from build123d import *

# Parameters (mm, degrees)
F1_DEPTH      = 25.4
F1_DEPTH_BACK = 25.4


with BuildPart() as f1:
    # F0 (on Front) → F1 (new body, two sides)
    with BuildSketch(Plane.XZ) as f1_sk:
        with BuildLine():
            Line((-8.390563, 22.175057), (-48.245732, 0))
            Line((-48.245732, 0), (-97.690113, -9.289551))
            Line((-97.690113, -9.289551), (-97.690113, -29.067304))
            Line((-97.690113, -29.067304), (-72.518431, -29.067304))
            ThreePointArc((-72.518431, -29.067304), (-57.08579, -12.585117), (-41.653149, -29.067304))
            Line((-41.653149, -29.067304), (38.356856, -29.067304))
            ThreePointArc((38.356856, -29.067304), (50.593399, -7.999803), (61.131231, -29.966293))
            Line((61.131231, -29.966293), (91.397189, -29.966293))
            Line((91.397189, -29.966293), (91.397189, -4.195281))
            Line((91.397189, -4.195281), (65.925851, 0))
            Line((65.925851, 0), (42.098479, 22.175057))
            Line((42.098479, 22.175057), (-8.390563, 22.175057))
        make_face()
    extrude(amount=F1_DEPTH)
    extrude(f1_sk.sketch, amount=-F1_DEPTH_BACK)


solid = f1.part
The listing builds one solid part. Answer for the finished solid, in the listing's coordinates (mm). A direction names the side the tool comes from. Give positions to 0.01 mm unless a question says otherwise; leave off trailing zeros. Loops run counter-clockwise (first coordinate to the right, second up) from the corner with the lowest first, then second, coordinate; pieces in that order, holes last. Notation, with made-up numbers: (13, -8.5) - (55, -8.5) arc R14 ccw to (55, 13.5) - close; hole circle Ø10 at (77, 31.5). An arc over 180 degrees is marked (long way). Answer as a JSON object with one key per item and string values.
1. Find the intervals of material crossed by L1, parallel to X at y = -9.5, z = -22; L2, parallel to X at y = -5, z = -23; L3, parallel to Z at x = 24, y = -13.5, in increasing order. Write a range as [from, to].
Determined:
{"L1": "[-97.69, -71.32], [-42.85, 36.27], [63.83, 91.4]", "L2": "[-97.69, -71.7], [-42.47, 36.32], [63.78, 91.4]", "L3": "[-29.07, 22.18]"}
2. A cutting plane is placed at D-D (z = 5). Write down the section's boundary in (x, y), then the cut area to 3 significant figures.
Determined:
{"outline": "(-39.26, -25.4) - (60.55, -25.4) - (60.55, 25.4) - (-39.26, 25.4) - close", "area": "5,070 mm²"}
3. A cutting plane is placed at A-A (z = -22). Write down the section's boundary in (x, y), then the cut area to 3 significant figures.
Determined:
{"outline": "(-97.69, -25.4) - (-71.32, -25.4) - (-71.32, 25.4) - (-97.69, 25.4) - close; (-42.85, -25.4) - (36.27, -25.4) - (36.27, 25.4) - (-42.85, 25.4) - close; (63.83, -25.4) - (91.4, -25.4) - (91.4, 25.4) - (63.83, 25.4) - close", "area": "6,760 mm²"}
4. For a pull along X with two mould halves and no side action, classify faces 3 (the flat face through (-4, -25.4, -9)), 4 (the flat face through (-28.04, -0.36, 11.24)), 5 (the cylindrical face through (-57.44, -0.36, -12.59)) as pulls with the +X half, pulls with the -X half, needs draft (parallel to the pull), parting line crosses it, or undercut.
Determined:
{"face 3": "needs draft", "face 4": "pulls with the -X half", "face 5": "undercut"}
5. Flat-ended cylindrical pins translate along their axes: pin 1 Ø8 at (x, y) = (-17, -1) entering from -Z; pin 2 Ø5 at (x, y) = (64, -7) entering from +Z; pin 3 Ø2 at (y, z) = (10, 6) entering from -X. Find the tip coordinate at first contact, or state that the pin passes through.
Determined:
{"pin 1": "z = -29.07", "pin 2": "z = 4.12", "pin 3": "x = -39.26"}
6. For faces 1 (the flat face through (-4, 25.4, -9)), 2 (the flat face through (-85, 0, -29.067)), determine the directions among +Z, -Z, +X, -X, +Y, -Y from which every point of the face is accessible in a straight line to the end or side of a thin tool.
Determined:
{"face 1": "+Z, -Z, +X, -X, +Y", "face 2": "-Z, -X, +Y, -Y"}
7. A cutting plane is placed at B-B (y = 9). Write down the section's boundary in (x, z), then the cut area to 3 significant figures.
Determined:
{"outline": "(-97.69, -29.07) - (-72.52, -29.07) arc R15.47 cw (long way) to (-41.65, -29.07) - (38.36, -29.07) arc R13.78 cw (long way) to (61.13, -29.97) - (91.4, -29.97) - (91.4, -4.2) - (65.93, 0) - (42.1, 22.18) - (-8.39, 22.18) - (-48.25, 0) - (-97.69, -9.29) - close", "area": "6,170 mm²"}
8. A cutting plane is placed at C-C (x = 12). Write down the section's boundary in (y, z).
Determined:
{"outline": "(-25.4, -29.07) - (25.4, -29.07) - (25.4, 22.18) - (-25.4, 22.18) - close"}
